Part model, mm, in its own coordinate system. A direction names the side the tool comes from. Round coordinates to 2 decimals unless told otherwise and drop trailing zeros. Write each loop counter-clockwise with the first axis right and the second up, starting at its lowest first coordinate (ties: lowest second). Pieces come first, ordered by that corner, then holes.
```python
from build123d import *

# Parameters (mm, degrees)
SKETCH1_W               = 203.2
SKETCH1_H               = 101.6
BOSS_EXTRUDE2_DEPTH     = 13.462
CUT_EXTRUDE1_DEPTH      = 13.208
CUT_EXTRUDE1_DEPTH_BACK = 28.448
SKETCH4_W               = 75
SKETCH4_H               = 23.376263875
SKETCH5_R               = 16.179381977
BOSS_EXTRUDE4_DEPTH     = 1.524
SKETCH6_R               = 8.05355352
BOSS_EXTRUDE6_DEPTH     = 11.43


with BuildPart() as part:
    # Sketch1 → Boss-Extrude2 (new body)
    with BuildSketch(Plane(origin=(0, 0, 0), x_dir=(1, 0, 0), z_dir=(0, 1, 0))):
        Rectangle(SKETCH1_W, SKETCH1_H)
    extrude(amount=BOSS_EXTRUDE2_DEPTH)

    # Sketch4 → Cut-Extrude1 (cut, two sides: drawn at the far end of the back side and taken through both)
    with BuildSketch(Plane(origin=(0, 13.462, 0), x_dir=(1, 0, 0), z_dir=(0, 1, 0)).offset(-CUT_EXTRUDE1_DEPTH_BACK)):
        with Locations((51.78549459, -45.778516755)):
            Rectangle(SKETCH4_W, SKETCH4_H)
        with Locations((51.78549459, 45.778516755)):
            Rectangle(SKETCH4_W, SKETCH4_H)
    extrude(amount=CUT_EXTRUDE1_DEPTH + CUT_EXTRUDE1_DEPTH_BACK, mode=Mode.SUBTRACT)

    # Sketch5 → Boss-Extrude4 (add)
    with BuildSketch(Plane(origin=(0, 0, 0), x_dir=(-1, 0, 0), z_dir=(0, -1, 0))):
        with Locations(Location((81.651405353, 0, 0), (0, 0, 270))):
            Circle(SKETCH5_R)
    extrude(amount=BOSS_EXTRUDE4_DEPTH)

    # Sketch6 → Boss-Extrude6 (add)
    with BuildSketch(Plane.XZ.offset(1.524)):
        with Locations(Location((-81.651405353, 0, 0), (0, 0, 270))):
            Circle(SKETCH6_R)
    extrude(amount=BOSS_EXTRUDE6_DEPTH)

    # Sketch7 → Revolve1 (revolve)
    with BuildSketch(Plane.XZ.offset(12.954)):
        with BuildLine():
            Line((-86.486836617, 0), (-76.815974088, 0))
            ThreePointArc((-76.815974088, 0), (-81.651405353, 4.835431264), (-86.486836617, 0))
        make_face()
    revolve(axis=Axis((-86.486836617, -12.954, 0), (1, 0, 0)))


solid = part.part
```
Q1. Cut at C-C on z = 0. Write the cut outline in (x, y).
Values follow:
outline: (-101.6, 0) - (-97.83, 0) - (-97.83, -1.52) - (-89.7, -1.52) - (-89.7, -12.95) - (-86.49, -12.95) arc R4.84 ccw to (-76.82, -12.95) - (-73.6, -12.95) - (-73.6, -1.52) - (-65.47, -1.52) - (-65.47, 0) - (101.6, 0) - (101.6, 13.46) - (-101.6, 13.46) - close
Q2. Which spindle directions (+Z, -Z, +X, -X, +Y, -Y) get a long thin tool onto all of the face, cutting with end or side? Do faces 1 (the flat face through (14.285, 7, 43)), 2 (the flat face through (51, 7, -34.09)), 3 (the flat face through (-89, -1.524, -4)). Say none if no direction does.
Values follow:
face 1: +Z, +Y, -Y
face 2: -Z, +Y, -Y
face 3: -Y
Q3. Wall check: L1, parallel to X at y = 6, z = -38.5; L2, parallel to Y at x = -36, z = 31.5; L3, parallel to Z at x = 51.5, y = 11. Give the ranges that are in metal, low to high.
Values follow:
L1: x = -101.6 to 14.29, 89.29 to 101.6
L2: y = 0 to 13.46
L3: z = -34.09 to 34.09
Q4. Cut at B-B on y = 5. Write the cut outline in (x, z).
Values follow:
outline: (-101.6, -50.8) - (14.29, -50.8) - (14.29, -34.09) - (89.29, -34.09) - (89.29, -50.8) - (101.6, -50.8) - (101.6, 50.8) - (89.29, 50.8) - (89.29, 34.09) - (14.29, 34.09) - (14.29, 50.8) - (-101.6, 50.8) - close
Q5. Cut at A-A on z = 42.5. Write the cut outline in (x, y).
Values follow:
outline: (-101.6, 0) - (14.29, 0) - (14.29, 13.46) - (-101.6, 13.46) - close; (89.29, 0) - (101.6, 0) - (101.6, 13.46) - (89.29, 13.46) - close
Q6. Mould opens along X. For faces 4 (the flat face through (-1, 13.462, -1)), 5 (the cylindrical face through (-97.693, -0.751, -2.106)), 6 (the flat face through (14.285, 7, -42)) say: +X half, -X half, draft (parallel to the pull), parting line (faces both ways), or undercut.
Values follow:
face 4: draft
face 5: parting line
face 6: undercut
Q7. Drop flat-ended pins along their axis: pin 1 (9.5 mm diameter, centred on x = -89, z = -5, fed in from -Y); pin 2 (17.5 mm diameter, centred on x = -82.5, z = 0, fed in from -Y); pin 3 (15 mm diameter, centred on x = 36.5, y = 3.5, fed in from -Z); pin 4 (6.5 mm diameter, centred on x = 49.5, y = 7, fed in from +Z). Give the stop position or say it passes through.
Values follow:
pin 1: stops at y = -15.46
pin 2: stops at y = -17.79
pin 3: stops at z = -34.09
pin 4: stops at z = 34.09
Q8. Cut at D-D on x = -43.5. Write the cut outline in (y, z).
Values follow:
outline: (0, -50.8) - (13.46, -50.8) - (13.46, 50.8) - (0, 50.8) - close
